Check sheet for the modelled part. Datum: model origin and axes. Units: mm. A direction names the side the tool comes from. Coordinates: 2 decimals unless noted, no trailing zeros. Loops run counter-clockwise (first coordinate to the right, second up) from the corner with the lowest first, then second, coordinate; pieces in that order, holes last. Notation, with made-up numbers: M 11,-33 L 16,-33 A20 cw 16,-29 Z; hole C -26,-21 d9. An arc over 180 degrees is marked long. Use CSV: the item, a comma, the result in double quotes. Start each with the question number.
(1) Go/stop test with a flat-tipped pin: pin 1 Ø1.5 at (x, y) = (14.5, -0.5) entering from +Z. Record where the tip stops, or that it passes through.
(2) Scan lines: line 1 (Y direction, x = 17, z = 5.5); line 2 (X direction, y = -12.75, z = 38); line 3 (Z direction, x = 0, y = -12.85). Record each from-to range of solid material in increasing order.
(3) Section check D-D on z = 35. Give the number of separate pieces and of enclosed holes in the cut face, and give its area (3 significant figures).
(4) Section check B-B on x = -29.5. Record the cut outline in (y, z).
(5) Section check A-A on y = -6.5. Record the cut outline in (x, z), and give its area (3 significant figures).
(6) Set-up check for faces 1 (the flat face through (-1, -12.5, 23)), 2 (the cylindrical face through (34.8, -13.5, 37.6)): record each of +Z, -Z, +X, -X, +Y, -Y from which the full face is reachable in a straight line by a thin tool's end or side.
(7) Section check C-C on z = 14.5. Record the cut outline in (x, y), and give its area (3 significant figures).
(8) Draft check along X on faces 3 (the cylindrical face through (0, 8, 1)), 4 (the cylindrical face through (0.63, -13.933, 0.598)). Enter one of: pulls with the +X half, pulls with the -X half, needs draft (parallel to the pull), parting line crosses it, or undercut.
from build123d import *

# Parameters (mm, degrees)
SKETCH_W        = 90
SKETCH_H        = 29
PAD_DEPTH       = 2
SKETCH001_W     = 90
SKETCH001_H     = 2
PAD001_DEPTH    = 42
FILLET_R        = 1.99
SKETCH002_R     = 4
SKETCH002_R_2   = 1.5
POCKET_DEPTH    = 29.001
SKETCH003_R     = 1.5
SKETCH003_R_2   = 4
POCKET001_DEPTH = 5
FILLET001_R     = 5


with BuildPart() as part:
    # Sketch → Pad (new body)
    with BuildSketch(Plane.XY):
        Rectangle(SKETCH_W, SKETCH_H)
    extrude(amount=PAD_DEPTH)

    # Sketch001 (on Face6 of Pad) → Pad001 (join)
    with BuildSketch(Plane.XY.offset(2)):
        with Locations((0, 13.5)):
            Rectangle(SKETCH001_W, SKETCH001_H)
        with Locations((0, -13.5)):
            Rectangle(SKETCH001_W, SKETCH001_H)
    extrude(amount=PAD001_DEPTH)

    # Fillet
    fillet_edges = [part.edges().sort_by_distance(p)[0] for p in [
        (0, 14.5, 0),
        (0, -14.5, 0),
    ]]
    fillet(fillet_edges, radius=FILLET_R)

    # Sketch002 (on Face15 of Fillet) → Pocket (cut, through all)
    with BuildSketch(Plane.XZ.offset(14.5)):
        with Locations((-36, 32)):
            Circle(SKETCH002_R)
        with Locations((-36, 38.5)):
            Circle(SKETCH002_R_2)
        with Locations((-29.5, 32)):
            Circle(SKETCH002_R_2)
        with Locations((-36, 25.5)):
            Circle(SKETCH002_R_2)
        with Locations((-42.5, 32)):
            Circle(SKETCH002_R_2)
        with Locations((36, 32)):
            Circle(SKETCH002_R)
        with Locations((36, 38.5)):
            Circle(SKETCH002_R_2)
        with Locations((29.5, 32)):
            Circle(SKETCH002_R_2)
        with Locations((36, 25.5)):
            Circle(SKETCH002_R_2)
        with Locations((42.5, 32)):
            Circle(SKETCH002_R_2)
        with Locations((0, 32)):
            Circle(SKETCH002_R)
        with Locations((0, 38.5)):
            Circle(SKETCH002_R_2)
        with Locations((6.5, 32)):
            Circle(SKETCH002_R_2)
        with Locations((0, 25.5)):
            Circle(SKETCH002_R_2)
        with Locations((-6.5, 32)):
            Circle(SKETCH002_R_2)
    extrude(amount=-POCKET_DEPTH, mode=Mode.SUBTRACT)

    # Sketch003 (on Face9 of Pocket) → Pocket001 (cut)
    with BuildSketch(Plane(origin=(0, 0, 0), x_dir=(1, 0, 0), z_dir=(0, 0, -1))):
        with Locations((-36, 6.5)):
            Circle(SKETCH003_R)
        with Locations((-36, 0)):
            Circle(SKETCH003_R_2)
        with Locations((-36, -6.5)):
            Circle(SKETCH003_R)
        with Locations((-29.5, 0)):
            Circle(SKETCH003_R)
        with Locations((-42.5, 0)):
            Circle(SKETCH003_R)
        with Locations((36, 6.5)):
            Circle(SKETCH003_R)
        with Locations((36, 0)):
            Circle(SKETCH003_R_2)
        with Locations((36, -6.5)):
            Circle(SKETCH003_R)
        with Locations((29.5, 0)):
            Circle(SKETCH003_R)
        with Locations((42.5, 0)):
            Circle(SKETCH003_R)
        with Locations((0, 6.5)):
            Circle(SKETCH003_R)
        Circle(SKETCH003_R_2)
        with Locations((0, -6.5)):
            Circle(SKETCH003_R)
        with Locations((6.5, 0)):
            Circle(SKETCH003_R)
        with Locations((-6.5, 0)):
            Circle(SKETCH003_R)
    extrude(amount=-POCKET001_DEPTH, mode=Mode.SUBTRACT)

    # Fillet001
    fillet001_edges = [part.edges().sort_by_distance(p)[0] for p in [
        (45, -13.5, 44),
        (45, 13.5, 44),
        (-45, 13.5, 44),
        (-45, -13.5, 44),
    ]]
    fillet(fillet001_edges, radius=FILLET001_R)


solid = part.part
Outcome:
1,pin 1,"stops at z = 2"
2,line 1,"y = -14.5 to -12.5, 12.5 to 14.5"
2,line 2,"x = -45 to -37.41, -34.59 to -1.41, 1.41 to 34.59, 37.41 to 45"
2,line 3,"z = 0.03 to 24, 27 to 28, 36 to 37, 40 to 44"
3,separate pieces,"8"
3,enclosed holes,"0"
3,area,"297 mm²"
4,outline,"M -14.5,1.99 A1.99 ccw -12.51,0 L -1.5,0 L -1.5,2 L -12.5,2 L -12.5,30.5 L -14.5,30.5 Z; M -14.5,33.5 L -12.5,33.5 L -12.5,44 L -14.5,44 Z; M 1.5,0 L 12.51,0 A1.99 ccw 14.5,1.99 L 14.5,30.5 L 12.5,30.5 L 12.5,2 L 1.5,2 Z; M 12.5,33.5 L 14.5,33.5 L 14.5,44 L 12.5,44 Z"
5,outline,"M -45,0 L -37.5,0 L -37.5,2 L -45,2 Z; M -34.5,0 L -1.5,0 L -1.5,2 L -34.5,2 Z; M 1.5,0 L 34.5,0 L 34.5,2 L 1.5,2 Z; M 37.5,0 L 45,0 L 45,2 L 37.5,2 Z"
5,area,"162 mm²"
6,face 1,"+Z, +X, -X"
6,face 2,"+Y, -Y"
7,outline,"M -45,-14.5 L 45,-14.5 L 45,-12.5 L -45,-12.5 Z; M -45,12.5 L 45,12.5 L 45,14.5 L -45,14.5 Z"
7,area,"360 mm²"
8,face 3,"undercut"
8,face 4,"needs draft"
